Read the model definition and answer for the solid it produces. Units are mm, in the model's axes. Face numbers are marked on the shaded views. A direction names the side the tool comes from. Coordinates: 2 decimals unless noted, no trailing zeros. Loops run counter-clockwise (first coordinate to the right, second up) from the corner with the lowest first, then second, coordinate; pieces in that order, holes last. Notation, with made-up numbers: M -9,67 L 16,67 A27 ccw 16,96 Z; hole C -2,-24 d6. An arc over 180 degrees is marked long. One line per item, written item: value. Start each with the question number.
```python
from build123d import *

# Parameters (mm, degrees)
SKETCH1_R               = 30
BOSS_EXTRUDE1_DEPTH     = 200
BOSS_EXTRUDE2_START     = -60
SKETCH2_R               = 4
BOSS_EXTRUDE2_DEPTH     = 80
BOSS_EXTRUDE3_DEPTH     = 10
BOSS_EXTRUDE4_DEPTH     = 10
FILLET1_R               = 10
FILLET2_R               = 3
CUT_EXTRUDE1_START      = -34
SKETCH7_R               = 4
CUT_EXTRUDE1_DEPTH      = 12
SKETCH8_R               = 2
CUT_EXTRUDE2_DEPTH      = 70
BOSS_EXTRUDE6_START     = 0.1
SKETCH9_R               = 2
BOSS_EXTRUDE6_DEPTH     = 70
CUT_EXTRUDE4_START      = -30
CUT_EXTRUDE4_DEPTH      = 35
SKETCH12_W              = 1
SKETCH12_H              = 2.4
CUT_EXTRUDE5_DEPTH      = 20
SKETCH14_R              = 30
CUT_EXTRUDE6_DEPTH      = 200
SKETCH15_R              = 97.689585443
SKETCH15_R_2            = 2
CUT_EXTRUDE7_DEPTH      = 200
SKETCH16_W              = 5.14946919
SKETCH16_H              = 11.525449866
CUT_EXTRUDE8_DEPTH      = 200
CUT_EXTRUDE8_DEPTH_BACK = 200
SKETCH17_W              = 4
SKETCH17_H              = 5
CUT_EXTRUDE9_DEPTH      = 200
CUT_EXTRUDE9_DEPTH_BACK = 200
SKETCH19_W              = 8.073982183
SKETCH19_H              = 13.216207409
CUT_EXTRUDE11_DEPTH     = 7
SKETCH20_W              = 16.90925267
SKETCH20_H              = 17.799092854
CUT_EXTRUDE12_DEPTH     = 3
SKETCH21_W              = 18.708797059
SKETCH21_H              = 16.020174298
CUT_EXTRUDE13_DEPTH     = 3
SKETCH22_W              = 8.604903729
SKETCH22_H              = 5.934872157
CUT_EXTRUDE14_DEPTH     = 30.73
CUT_EXTRUDE15_DEPTH     = 5
SKETCH24_R              = 2
SKETCH24_R_2            = 1.95
CUT_EXTRUDE16_DEPTH     = 25


with BuildPart() as part:
    # Sketch1 → Boss-Extrude1 (new body)
    with BuildSketch(Plane(origin=(0, 0, 0), x_dir=(1, 0, 0), z_dir=(0, 1, 0))):
        Circle(SKETCH1_R)
    extrude(amount=BOSS_EXTRUDE1_DEPTH)

    # Sketch14 → Cut-Extrude6 (cut)
    with BuildSketch(Plane(origin=(0, 200, 0), x_dir=(1, 0, 0), z_dir=(0, 1, 0))):
        Circle(SKETCH14_R)
    extrude(amount=-CUT_EXTRUDE6_DEPTH, mode=Mode.SUBTRACT)


with BuildPart() as body_2:
    # Sketch2 → Boss-Extrude2 (new body)
    with BuildSketch(Plane(origin=(0, 200, 0), x_dir=(1, 0, 0), z_dir=(0, 1, 0)).offset(BOSS_EXTRUDE2_START)):
        with Locations((0, -50)):
            Circle(SKETCH2_R)
    extrude(amount=-BOSS_EXTRUDE2_DEPTH)

    # Sketch4 → Boss-Extrude3 (add)
    with BuildSketch(Plane(origin=(0, 140, 0), x_dir=(1, 0, 0), z_dir=(0, 1, 0))):
        with BuildLine():
            Line((-2.932848445, -47.28), (40.915854419, 0))
            Line((40.915854419, 0), (6, 37.648128431))
            Line((6, 37.648128431), (11.86569689, 43.088128431))
            Line((11.86569689, 43.088128431), (51.826748931, 0))
            Line((51.826748931, 0), (2.932848445, -52.72))
            ThreePointArc((2.932848445, -52.72), (2.72, -47.067151555), (-2.932848445, -47.28))
        make_face()
    extrude(amount=-BOSS_EXTRUDE3_DEPTH)

    # Sketch5 → Boss-Extrude4 (add)
    with BuildSketch(Plane.XZ.offset(-60)):
        with BuildLine():
            Line((6, -37.648128431), (11.86569689, -43.088128431))
            Line((11.86569689, -43.088128431), (51.826748931, 0))
            Line((51.826748931, 0), (2.932848445, 52.72))
            ThreePointArc((2.932848445, 52.72), (2.72, 47.067151555), (-2.932848445, 47.28))
            Line((-2.932848445, 47.28), (40.915854419, 0))
            Line((40.915854419, 0), (6, -37.648128431))
        make_face()
    extrude(amount=-BOSS_EXTRUDE4_DEPTH)

    # Fillet1
    fillet1_edges = [body_2.edges().sort_by_distance(p)[0] for p in [
        (40.915854419, 65, 0),
        (51.826748931, 65, 0),
        (40.915854419, 135, 0),
        (51.826748931, 135, 0),
    ]]
    fillet(fillet1_edges, radius=FILLET1_R)

    # Fillet2
    fillet2_edges = [body_2.edges().sort_by_distance(p)[0] for p in [
        (8.932848445, 140, -40.368128431),
        (6, 65, -37.648128431),
        (8.932848445, 70, -40.368128431),
        (11.86569689, 65, -43.088128431),
        (8.932848445, 60, -40.368128431),
        (8.932848445, 130, -40.368128431),
        (6, 135, -37.648128431),
        (11.86569689, 135, -43.088128431),
    ]]
    fillet(fillet2_edges, radius=FILLET2_R)

    # Sketch7 → Cut-Extrude1 (cut)
    with BuildSketch(Plane(origin=(0, 140, 0), x_dir=(1, 0, 0), z_dir=(0, 1, 0)).offset(CUT_EXTRUDE1_START)):
        with Locations((0, -50)):
            Circle(SKETCH7_R)
    extrude(amount=-CUT_EXTRUDE1_DEPTH, mode=Mode.SUBTRACT)

    # Sketch8 → Cut-Extrude2 (cut)
    with BuildSketch(Plane(origin=(0, 140, 0), x_dir=(1, 0, 0), z_dir=(0, 1, 0))):
        with Locations((0, -50)):
            Circle(SKETCH8_R)
    extrude(amount=-CUT_EXTRUDE2_DEPTH, mode=Mode.SUBTRACT)

    # Sketch9 → Boss-Extrude6 (add)
    with BuildSketch(Plane(origin=(0, 140, 0), x_dir=(1, 0, 0), z_dir=(0, 1, 0)).offset(BOSS_EXTRUDE6_START)):
        with Locations((0, -50)):
            Circle(SKETCH9_R)
    extrude(amount=-BOSS_EXTRUDE6_DEPTH)

    # Sketch11 → Cut-Extrude4 (cut)
    with BuildSketch(Plane(origin=(0, 140.1, 0), x_dir=(1, 0, 0), z_dir=(0, 1, 0)).offset(CUT_EXTRUDE4_START)):
        with BuildLine():
            Line((-0.975, -51.746245974), (-0.975, -48.253754026))
            ThreePointArc((-0.975, -48.253754026), (-2, -50), (-0.975, -51.746245974))
        make_face()
        with BuildLine():
            Line((0.975, -48.253754026), (0.975, -51.746245974))
            ThreePointArc((0.975, -51.746245974), (2, -50), (0.975, -48.253754026))
        make_face()
    extrude(amount=-CUT_EXTRUDE4_DEPTH, mode=Mode.SUBTRACT)

    # Sketch12 → Cut-Extrude5 (cut)
    with BuildSketch(Plane(origin=(0, 140.1, 0), x_dir=(1, 0, 0), z_dir=(0, 1, 0))):
        with Locations((0, -50)):
            Rectangle(SKETCH12_W, SKETCH12_H)
    extrude(amount=-CUT_EXTRUDE5_DEPTH, mode=Mode.SUBTRACT)

    # Sketch15 → Cut-Extrude7 (cut)
    with BuildSketch(Plane(origin=(0, 140, 0), x_dir=(1, 0, 0), z_dir=(0, 1, 0))):
        with Locations((0, -50)):
            Circle(SKETCH15_R)
        with BuildLine():
            Line((45.520251903, 6.8), (13.90569689, 40.888492097))
            Line((13.90569689, 40.888492097), (8.04, 35.448492097))
            Line((8.04, 35.448492097), (34.609357391, 6.8))
            ThreePointArc((34.609357391, 6.8), (37.277236279, 0), (34.609357391, -6.8))
            Line((34.609357391, -6.8), (-2.932848445, -47.28))
            ThreePointArc((-2.932848445, -47.28), (-2.72, -52.932848445), (2.932848445, -52.72))
            Line((2.932848445, -52.72), (45.520251903, -6.8))
            ThreePointArc((45.520251903, -6.8), (48.188130791, 0), (45.520251903, 6.8))
        make_face(mode=Mode.SUBTRACT)
        with BuildLine():
            ThreePointArc((45.520251903, -6.8), (48.188130791, 0), (45.520251903, 6.8))
            Line((45.520251903, 6.8), (13.90569689, 40.888492097))
            Line((13.90569689, 40.888492097), (8.04, 35.448492097))
            Line((8.04, 35.448492097), (34.609357391, 6.8))
            ThreePointArc((34.609357391, 6.8), (37.277236279, 0), (34.609357391, -6.8))
            Line((34.609357391, -6.8), (-2.932848445, -47.28))
            ThreePointArc((-2.932848445, -47.28), (-2.72, -52.932848445), (2.932848445, -52.72))
            Line((2.932848445, -52.72), (45.520251903, -6.8))
        make_face()
        with Locations((0, -50)):
            Circle(SKETCH15_R_2, mode=Mode.SUBTRACT)
    extrude(amount=-CUT_EXTRUDE7_DEPTH, mode=Mode.SUBTRACT)

    # Sketch16 → Cut-Extrude8 (cut, two sides)
    with BuildSketch(Plane(origin=(0.975, 0, 0), x_dir=(0, 0, -1), z_dir=(1, 0, 0))) as cut_extrude8_sk:
        with Locations((-49.425265405, 64.237275067)):
            Rectangle(SKETCH16_W, SKETCH16_H)
    extrude(amount=CUT_EXTRUDE8_DEPTH, mode=Mode.SUBTRACT)
    extrude(cut_extrude8_sk.sketch, amount=-CUT_EXTRUDE8_DEPTH_BACK, mode=Mode.SUBTRACT)

    # Sketch17 → Cut-Extrude9 (cut, two sides)
    with BuildSketch(Plane.ZY.offset(0.975)) as cut_extrude9_sk:
        with Locations((50, 72.6)):
            Rectangle(SKETCH17_W, SKETCH17_H)
    extrude(amount=CUT_EXTRUDE9_DEPTH, mode=Mode.SUBTRACT)
    extrude(cut_extrude9_sk.sketch, amount=-CUT_EXTRUDE9_DEPTH_BACK, mode=Mode.SUBTRACT)

    # Sketch19 → Cut-Extrude11 (cut)
    with BuildSketch(Plane(origin=(0, 140.1, 0), x_dir=(1, 0, 0), z_dir=(0, 1, 0))):
        with Locations((-1.711492601, -47.464499481)):
            Rectangle(SKETCH19_W, SKETCH19_H)
    extrude(amount=-CUT_EXTRUDE11_DEPTH, mode=Mode.SUBTRACT)

    # Sketch20 → Cut-Extrude12 (cut)
    with BuildSketch(Plane(origin=(0, 133.1, 0), x_dir=(1, 0, 0), z_dir=(0, 1, 0))):
        with Locations((1.357922153, -50.543868256)):
            Rectangle(SKETCH20_W, SKETCH20_H)
    extrude(amount=-CUT_EXTRUDE12_DEPTH, mode=Mode.SUBTRACT)

    # Sketch21 → Cut-Extrude13 (cut)
    with BuildSketch(Plane.XZ.offset(-75.1)):
        with Locations((-2.026585117, 52.503315088)):
            Rectangle(SKETCH21_W, SKETCH21_H)
    extrude(amount=-CUT_EXTRUDE13_DEPTH, mode=Mode.SUBTRACT)

    # Sketch22 → Cut-Extrude14 (cut)
    with BuildSketch(Plane.XZ.offset(-78.1)):
        with Locations((0.059480902, 50.237923606)):
            Rectangle(SKETCH22_W, SKETCH22_H)
    extrude(amount=-CUT_EXTRUDE14_DEPTH, mode=Mode.SUBTRACT)

    # Sketch23 → Cut-Extrude15 (cut)
    with BuildSketch(Plane.XZ.offset(-110.1)):
        with BuildLine():
            Line((-0.975, 51.746245974), (-0.975, 48.253754026))
            ThreePointArc((-0.975, 48.253754026), (-2, 50), (-0.975, 51.746245974))
        make_face()
        with BuildLine():
            Line((0.975, 48.253754026), (0.975, 51.746245974))
            ThreePointArc((0.975, 51.746245974), (2, 50), (0.975, 48.253754026))
        make_face()
    extrude(amount=-CUT_EXTRUDE15_DEPTH, mode=Mode.SUBTRACT)

    # Sketch24 → Cut-Extrude16 (cut)
    with BuildSketch(Plane(origin=(0, 130.1, 0), x_dir=(1, 0, 0), z_dir=(0, 1, 0))):
        with Locations((0, -50)):
            Circle(SKETCH24_R)
        with Locations((0, -50)):
            Circle(SKETCH24_R_2, mode=Mode.SUBTRACT)
    extrude(amount=-CUT_EXTRUDE16_DEPTH, mode=Mode.SUBTRACT)


solid = body_2.part
```
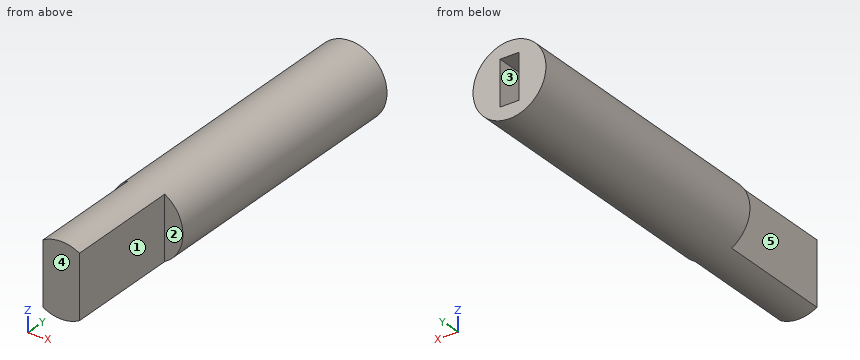
1) Section A-A (z = 50) is taken. Determine the outline of the cut face in (x, y) (3 decimals), then the cut area to 3 significant figures.
2) Section D-D (y = 116) is taken. Determine the outline of the cut face in (x, z).
3) Section C-C (y = 123.5) is taken. Determine the outline of the cut face in (x, z), then the cut area to 3 significant figures.
4) For a pull along X with two mould halves and no side action, classify the marked faces 1, 2 and 3 as released by +X, released by -X, zero draft, split by the parting line, or undercut.
5) A tool of negligible diameter and unlimited length cuts with its end or side. For the marked faces 4 and 5, from which of +Z, -Z, +X, -X, +Y, -Y can it reach the whole face along a straight path? Write none if from no direction.
6) Section B-B (x = 0) is taken. Determine the outline of the cut face in (y, z).
7) Flat-ended cylindrical pins translate along their axes: pin 1 (0.8 mm diameter, centred on x = 0, z = 50, fed in from +Y); pin 2 (1 mm diameter, centred on y = 110.5, z = 50, fed in from -X) (3 decimals); pin 3 (0.5 mm diameter, centred on x = -1.5, z = 50.5, fed in from -Y). Find the tip coordinate at first contact, or state that the pin passes through.
8) Consider line 1 along X through (y, z) = (127.75, 49.95); line 2 along Z through (x, y) = (-0.05, 120.5); line 3 along Y through (x, z) = (0.1, 49.4). Determine where each line is inside the solid, lowest interval first.
Results found:
1. outline: M -1.95,115.1 L -0.975,115.1 L -0.975,108.83 L 0.975,108.83 L 0.975,115.1 L 1.95,115.1 L 1.95,130.1 L 0.5,130.1 L 0.5,120.1 L -0.5,120.1 L -0.5,130.1 L -1.95,130.1 Z
1. area: 60.7 mm²
2. outline: C 0,50 d3.9
3. outline: C 0,50 d3.9; hole M -0.5,48.8 L 0.5,48.8 L 0.5,51.2 L -0.5,51.2 Z
3. area: 9.55 mm²
4. face 1: released by +X
4. face 2: zero draft
4. face 3: undercut
5. face 4: +Z, -Z, +X, -X, -Y
5. face 5: +Z, -Z, -X, -Y
6. outline: M 108.83,48.05 L 130.1,48.05 L 130.1,48.8 L 120.1,48.8 L 120.1,51.2 L 130.1,51.2 L 130.1,51.95 L 108.83,51.95 Z
7. pin 1: stops at y = 120.1
7. pin 2: stops at x = -0.975
7. pin 3: stops at y = 115.1
8. line 1: x = -1.95 to -0.5, 0.5 to 1.95
8. line 2: z = 48.05 to 48.8, 51.2 to 51.95
8. line 3: y = 108.83 to 120.1
